Answer from the drawing. Dimensions are ordinates in mm from the lowest x, y and z of the part. Coordinates: 2 decimals unless noted, no trailing zeros. Order: outer loops, then holes, each group sorted by start corner. A loop starts at its lowest first (then second) coordinate and runs counter-clockwise, first axis right, second up.
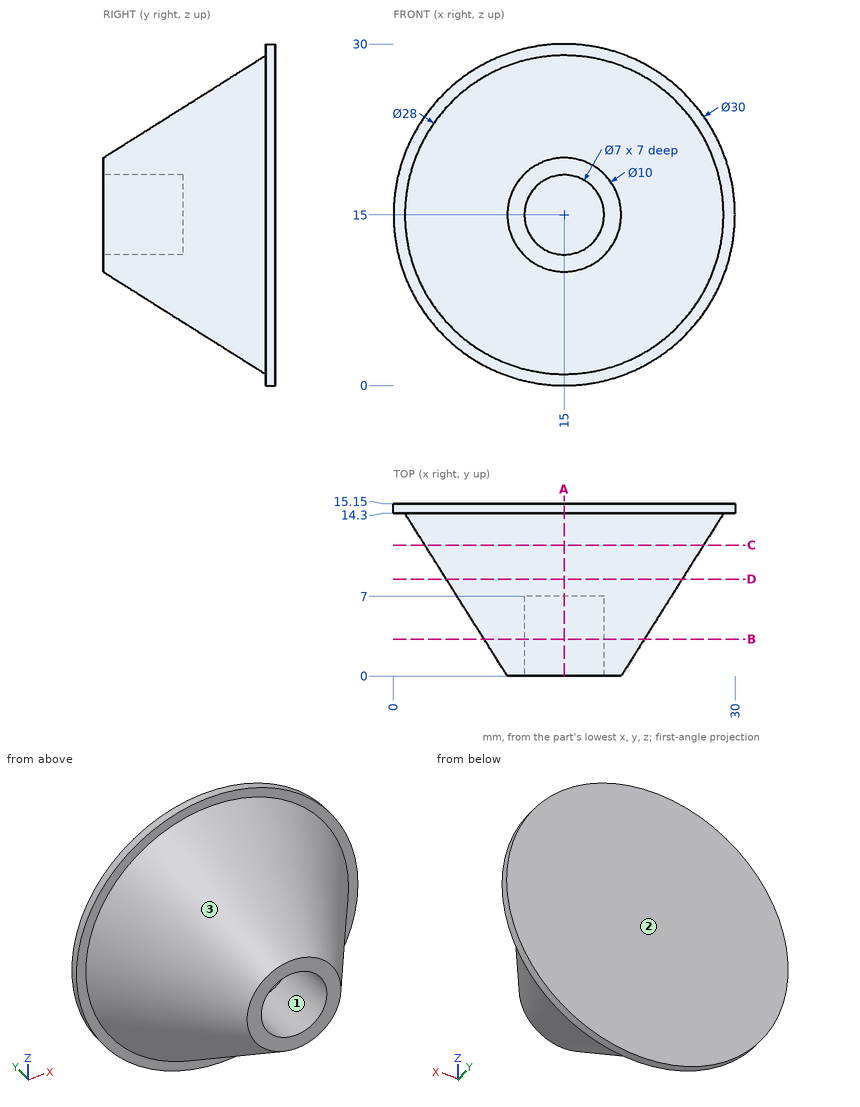
1. The part is cut by section A-A (x = 15). Determine the outline of the cut face in (y, z).
2. Consider probe 1 along Y at (x, z) = (11.75, 16); probe 2 along Z at (x, y) = (15, 4.5); probe 3 along Y at (x, z) = (21.25, 28.25). Determine where each line is inside the solid, lowest interval first.
3. The part is cut by section C-C (y = 11.5). Determine the outline of the cut face in (x, z), plus the area to 3 significant figures.
4. The mould has two halves that part along Z. Classify the marked faces 1, 2 and 3: released by +Z, released by -Z, zero draft, split by the parting line, or undercut.
5. Flat-ended cylindrical pins translate along their axes: pin 1 (1 mm diameter, centred on y = 2.5, z = 21, fed in from +X); pin 2 (2 mm diameter, centred on x = 8.5, y = 3.5, fed in from +Z); pin 3 (8 mm diameter, centred on x = 9, y = 6.5, fed in from +Z); pin 4 (3 mm diameter, centred on x = 25, y = 4, fed in from -Z). Find the tip coordinate at first contact, or state that the pin passes through.
6. The part is cut by section B-B (y = 3.25). Determine the outline of the cut face in (x, z), plus the area to 3 significant figures.
7. The part is cut by section D-D (y = 8.5). Determine the outline of the cut face in (x, z).
Worked out:
1. outline: (0, 10) - (14.3, 1) - (14.3, 0) - (15.15, 0) - (15.15, 30) - (14.3, 30) - (14.3, 29) - (0, 20) - (0, 18.5) - (7, 18.5) - (7, 11.5) - (0, 11.5) - close
2. probe 1: y = 7 to 15.15
2. probe 2: z = 7.17 to 11.5, 18.5 to 22.83
2. probe 3: y = 14.3 to 15.15
3. outline: circle Ø24.48 at (15, 15)
3. area: 470 mm2
4. face 1: undercut
4. face 2: zero draft
4. face 3: split by the parting line
5. pin 1: stops at x = 18.79
5. pin 2: stops at z = 20
5. pin 3: stops at z = 25.54
5. pin 4: passes through
6. outline: circle Ø14.09 at (15, 15); hole circle Ø7 at (15, 15)
6. area: 117 mm2
7. outline: circle Ø20.7 at (15, 15)
